Part print with two shaded views. Sizes in mm from the minimum x, y, z corner. Round coordinates to 2 decimals unless told otherwise and drop trailing zeros. Write each loop counter-clockwise with the first axis right and the second up, starting at its lowest first coordinate (ties: lowest second). Pieces come first, ordered by that corner, then holes. Notation, with made-up numbers: (16, -6) -> (23, -6) arc R11 cw to (23, 10) -> close; hole circle Ø1 at (-31, 39). An arc over 180 degrees is marked (long way). Put each result on its own line as item: value. Start each with the question number.
1. Drill centre lines: line 1 (X direction, y = 0.85, z = 203.2) (3 decimals); line 2 (Z direction, x = 63.5, y = 2.15) (3 decimals); line 3 (X direction, y = 1.6, z = 107.95). Where is each one in solid material? Low to high. Write a range as from..to.
2. Saw through at A-A on x = 63.5. List the corners of the cut face in (y, z) (3 decimals), and give its area (3 significant figures).
3. Saw through at D-D on y = 1.7. State how many separate pieces and enclosed holes the cut face has, and give its area (3 significant figures).
4. Flat gauge pin, fed straight in: P1, Ø5, axis at x = 12.7, z = 203.2, coming from the -Y side. Where does the tip first touch, or does it go through?
5. Saw through at C-C on x = 38.1. List the corners of the cut face in (y, z) (1 decimal), and give its area (3 significant figures).
6. Saw through at B-B on z = 12.7. List the corners of the cut face in (x, y) (3 decimals).
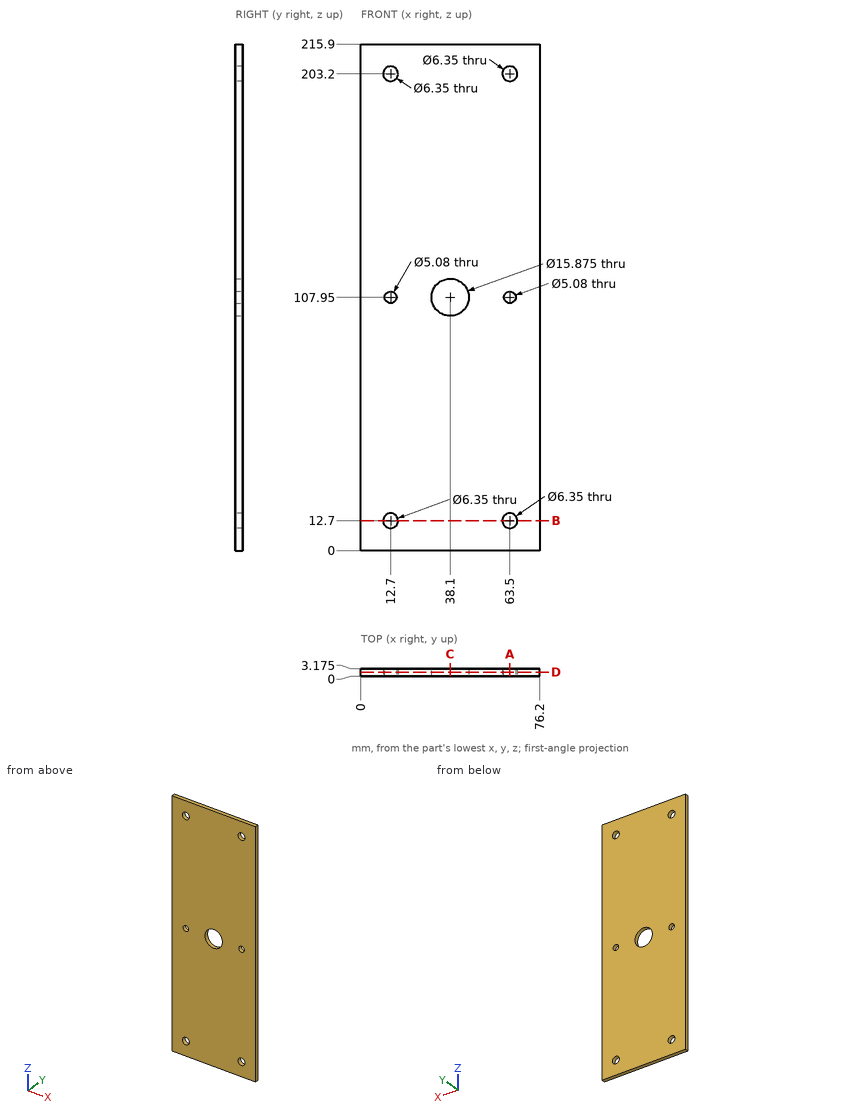
Return value:
1. line 1: x = 0..9.525, 15.875..60.325, 66.675..76.2
1. line 2: z = 0..9.525, 15.875..105.41, 110.49..200.025, 206.375..215.9
1. line 3: x = 0..10.16, 15.24..30.16, 46.04..60.96, 66.04..76.2
2. outline: (0, 0) -> (3.175, 0) -> (3.175, 9.525) -> (0, 9.525) -> close; (0, 15.875) -> (3.175, 15.875) -> (3.175, 105.41) -> (0, 105.41) -> close; (0, 110.49) -> (3.175, 110.49) -> (3.175, 200.025) -> (0, 200.025) -> close; (0, 206.375) -> (3.175, 206.375) -> (3.175, 215.9) -> (0, 215.9) -> close
2. area: 629 mm^2
3. separate pieces: 1
3. enclosed holes: 7
3. area: 16,100 mm^2
4. P1: passes through
5. outline: (0, 0) -> (3.2, 0) -> (3.2, 100) -> (0, 100) -> close; (0, 115.9) -> (3.2, 115.9) -> (3.2, 215.9) -> (0, 215.9) -> close
5. area: 635 mm^2
6. outline: (0, 0) -> (9.525, 0) -> (9.525, 3.175) -> (0, 3.175) -> close; (15.875, 0) -> (60.325, 0) -> (60.325, 3.175) -> (15.875, 3.175) -> close; (66.675, 0) -> (76.2, 0) -> (76.2, 3.175) -> (66.675, 3.175) -> close
